For this review, take the finished solid that the model builds, in its own axes (mm). Give positions to 0.01 mm unless a question says otherwise; leave off trailing zeros. Write each loop counter-clockwise with the first axis right and the second up, starting at its lowest first coordinate (ties: lowest second). Pieces come first, ordered by that corner, then holes.
from build123d import *

# Parameters (mm, degrees)
SKETCH1_R               = 58.499168585
BOSS_EXTRUDE1_DEPTH     = 95
CUT_EXTRUDE3_DEPTH      = 100
SKETCH4_W               = 9.373072574
SKETCH4_H               = 2.086863183
SKETCH4_W_2             = 2.476243421
SKETCH4_H_2             = 12.533404649
CUT_EXTRUDE4_DEPTH      = 127.730498931
SKETCH5_R               = 85.185879132
SKETCH5_R_2             = 48.091620782
CUT_EXTRUDE6_DEPTH      = 162.424468201
CUT_EXTRUDE9_DEPTH      = 123.740942834
CUT_EXTRUDE9_DEPTH_BACK = 123.740942834
SKETCH6_R               = 79.179320002
SKETCH6_R_2             = 47.965553318
SKETCH7_R               = 65.670207134
SKETCH7_R_2             = 49.501482781
CUT_EXTRUDE11_DEPTH     = 100


with BuildPart() as part:
    # Sketch1 → Boss-Extrude1 (new body)
    with BuildSketch(Plane(origin=(0, 0, 0), x_dir=(0, 0, -1), z_dir=(1, 0, 0))):
        with Locations((-1.612948614, 0)):
            Circle(SKETCH1_R)
    extrude(amount=BOSS_EXTRUDE1_DEPTH)

    # Sketch2 → Cut-Extrude3 (cut)
    with BuildSketch(Plane.ZY):
        Polygon((-34.616587509, 50.080454684), (-34.616587509, 62.895572105), (-0.820688819, 58.448525507), (0, 3.58366071), (-34.293670433, 46.428785299), align=None)
        with BuildLine():
            Line((-37.468242519, 43.529452383), (-2.046271026, 0.817665198))
            Line((-2.046271026, 0.817665198), (-56.886219972, 0))
            add(Edge.make_bspline(
                [(-37.468242519, 43.529452383), (-81.726208007, 46.47230528), (-56.886219972, 0)],
                knots=[0, 0, 0, 1, 1, 1], degree=2))
        make_face()
        with BuildLine():
            Line((-56.773526724, -3.629355702), (-2.046271026, -1.930047978))
            Line((-2.046271026, -1.930047978), (-45.251031563, -35.013141635))
            add(Edge.make_bspline(
                [(-56.773526724, -3.629355702), (-82.637840847, -33.762491691), (-45.251031563, -35.013141635)],
                knots=[0, 0, 0, 1, 1, 1], degree=2))
        make_face()
        with BuildLine():
            Line((-42.78323994, -38.093715585), (0.600944507, -2.836333045))
            Line((0.600944507, -2.836333045), (0, -58.476928116))
            add(Edge.make_bspline(
                [(-42.78323994, -38.093715585), (-42.157907188, -81.245363376), (0, -58.476928116)],
                knots=[0, 0, 0, 1, 1, 1], degree=2))
        make_face()
        with BuildLine():
            Line((3.225897227, -58.476928116), (2.505757473, -1.930047978))
            Line((2.505757473, -1.930047978), (37.676550811, -46.060496325))
            add(Edge.make_bspline(
                [(37.676550811, -46.060496325), (44.967631713, -79.6133954), (3.225897227, -58.476928116)],
                knots=[0, 0, 0, 1, 1, 1], degree=2))
        make_face()
        with BuildLine():
            Line((42.352672899, -41.981276663), (4.046586047, -0.931979638))
            Line((4.046586047, -0.931979638), (60.080269742, -1.930047978))
            add(Edge.make_bspline(
                [(60.080269742, -1.930047978), (94.049932739, -36.726987631), (42.352672899, -41.981276663)],
                knots=[0, 0, 0, 1, 1, 1], degree=2))
        make_face()
        with BuildLine():
            Line((60.080269742, 1.930047978), (4.046586047, 1.930047978))
            Line((4.046586047, 1.930047978), (51.077950448, 31.230855234))
            add(Edge.make_bspline(
                [(51.077950448, 31.230855234), (102.146773926, 32.028777375), (60.080269742, 1.930047978)],
                knots=[0, 0, 0, 1, 1, 1], degree=2))
        make_face()
        with BuildLine():
            Line((48.248640535, 35.316638631), (2.505757473, 3.58366071))
            Line((2.505757473, 3.58366071), (4.046586047, 58.448525507))
            add(Edge.make_bspline(
                [(4.046586047, 58.448525507), (39.246107014, 77.741383534), (48.248640535, 35.316638631)],
                knots=[0, 0, 0, 1, 1, 1], degree=2))
        make_face()
    extrude(amount=-CUT_EXTRUDE3_DEPTH, mode=Mode.SUBTRACT)

    # Sketch4 → Cut-Extrude4 (cut, through all)
    with BuildSketch(Plane.ZY):
        with Locations((2.834262756, 59.310645652)):
            Rectangle(SKETCH4_W, SKETCH4_H)
        with Locations((-57.79093587, -1.746234162)):
            Rectangle(SKETCH4_W_2, SKETCH4_H_2)
    extrude(amount=-CUT_EXTRUDE4_DEPTH, mode=Mode.SUBTRACT)

    # Sketch5 → Cut-Extrude6 (cut, through all)
    with BuildSketch(Plane(origin=(0, 0, -56.552814159), x_dir=(-1, 0, 0), z_dir=(0, 0, -1))):
        with Locations((-47.078327147, -2.012615685)):
            Circle(SKETCH5_R)
        with Locations((-47.078327147, -2.012615685)):
            Circle(SKETCH5_R_2, mode=Mode.SUBTRACT)
    extrude(amount=-CUT_EXTRUDE6_DEPTH, mode=Mode.SUBTRACT)

    # Sketch6 → Cut-Extrude9 (cut, two sides: drawn at the far end of the back side and taken through both)
    with BuildSketch(Plane(origin=(0, -0.859629379, -0.015311663), x_dir=(-1, 0, 0), z_dir=(0, -0.9998414052195305, -0.017809110270727707)).offset(-CUT_EXTRUDE9_DEPTH_BACK)):
        with Locations((-47.673789364, -1.454840891)):
            Circle(SKETCH6_R)
        with Locations((-47.673789364, -1.454840891)):
            Circle(SKETCH6_R_2, mode=Mode.SUBTRACT)
    extrude(amount=CUT_EXTRUDE9_DEPTH + CUT_EXTRUDE9_DEPTH_BACK, mode=Mode.SUBTRACT)

    # Sketch7 → Cut-Extrude11 (cut)
    with BuildSketch(Plane(origin=(95, 0, 0), x_dir=(0, 0, -1), z_dir=(1, 0, 0))):
        with Locations((-2.505757473, -1.930047978)):
            Circle(SKETCH7_R)
        with Locations((-2.505757473, -1.930047978)):
            Circle(SKETCH7_R_2, mode=Mode.SUBTRACT)
    extrude(amount=-CUT_EXTRUDE11_DEPTH, mode=Mode.SUBTRACT)


solid = part.part
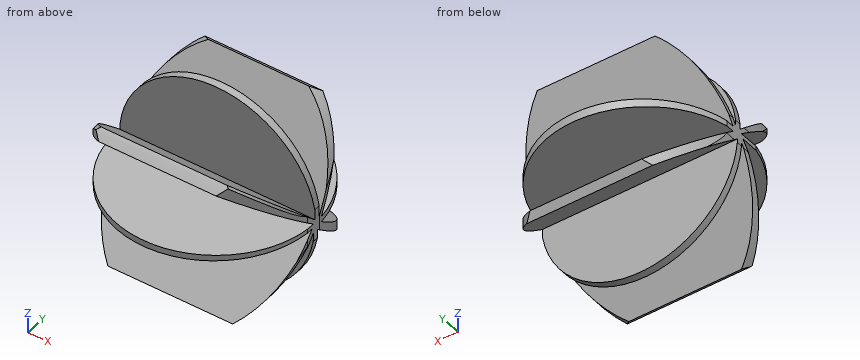
(1) We need section B-B (y = -16). Count the separate pieces of the cut face and the enclosed holes in it, and give its area (3 significant figures).
(2) We need section D-D (x = 65.5). Write out the cut boundary in (y, z), and give its area (3 significant figures).
(3) We need section A-A (x = 46.5). Write out the cut boundary in (y, z), and give its area (3 significant figures).
(4) For L1, parallel to Z at x = 71, y = 19; L2, parallel to Y at x = 86, z = -4; L3, parallel to Z at x = 83.5, y = 6, list the stretches that pass through material, from the lowest coordinate up.
(5) Clearance check with flat-ended pins moving along their axes: pin 1 Ø12 at (x, y) = (13.5, 22.5) entering from -Z; pin 2 Ø10 at (x, y) = (74, -14.5) entering from +Z; pin 3 Ø8 at (x, y) = (37, 1.5) entering from -Z. State where each tip first meets the part, or that it passes through.
The answers:
1. separate pieces: 3
1. enclosed holes: 0
1. area: 1,030 mm2
2. outline: (-46.44, 0.13) - (-2.84, 0.6) - (-32.76, -36.22) arc R49.5 ccw to (-29.78, -38.42) - (-1.93, -2.05) - (-3.21, -43.14) - (0.21, -43.08) - (0.82, -2.05) - (35.03, -30.42) arc R49.5 ccw to (37.63, -27.25) - (3.58, 0) - (42.41, -0.58) - (42.41, 3.6) - (3.58, 2.51) - (29.89, 40.43) arc R49.5 ccw to (26.3, 43.17) - (1.93, 4.05) - (1.93, 46.03) - (-1.68, 45.96) - (-0.93, 4.05) - (-36.86, 37.58) arc R49.5 ccw to (-40.64, 33.36) - (-1.93, 2.51) - (-46.44, 3.07) - close
2. area: 1,170 mm2
3. outline: (-50.1, 0.09) - (-2.84, 0.6) - (-32.76, -36.22) arc R49.5 ccw to (-29.78, -38.42) - (-1.93, -2.05) - (-3.31, -46.56) - (0.15, -46.5) - (0.82, -2.05) - (35.03, -30.42) arc R49.5 ccw to (37.63, -27.25) - (3.58, 0) - (46.08, -0.64) - (46.08, 3.7) - (3.58, 2.51) - (29.89, 40.43) arc R49.5 ccw to (26.3, 43.17) - (1.93, 4.05) - (1.93, 49.45) - (-1.74, 49.38) - (-0.93, 4.05) - (-36.86, 37.58) arc R49.5 ccw to (-40.64, 33.36) - (-1.93, 2.51) - (-50.1, 3.12) - close
3. area: 1,230 mm2
4. L1: z = -17.13 to -12.34, -0.23 to 2.94, 24.73 to 31.45
4. L2: y = -6.58 to -3.43, -1.99 to 0.79, 3.17 to 8.58
4. L3: z = -6.34 to -1.93, -0.04 to 2.57, 5.99 to 10.58
5. pin 1: stops at z = -25
5. pin 2: stops at z = 21.37
5. pin 3: stops at z = -46.02
